Here's how the part is built. I have some questions about the finished solid (model axes, mm). Coordinates: 2 decimals unless noted, no trailing zeros. Order: outer loops, then holes, each group sorted by start corner. A loop starts at its lowest first (then second) coordinate and runs counter-clockwise, first axis right, second up.
```python
from build123d import *

# Parameters (mm, degrees)
SKETCH1_W           = 3.3
SKETCH1_H           = 3
SKETCH1_W_2         = 3
SKETCH1_H_2         = 3.3
BOSS_EXTRUDE1_DEPTH = 3


with BuildPart() as part:
    # Sketch1 → Boss-Extrude1 (new body)
    with BuildSketch(Plane.XY):
        Polygon((165, 252), (156, 243), (120, 243), (111, 252), (111, 288), (120, 297), (156, 297), (165, 288), align=None)
        with Locations((117.15, 254.994383568)):
            Rectangle(SKETCH1_W, SKETCH1_H, mode=Mode.SUBTRACT)
        Polygon((136.5, 274.5), (136.5, 271.5), (133.5, 271.5), (133.5, 268.5), (136.5, 268.5), (136.5, 265.5), (139.5, 265.5), (139.5, 268.5), (142.5, 268.5), (142.5, 271.5), (139.5, 271.5), (139.5, 274.5), align=None, mode=Mode.SUBTRACT)
        with Locations((117.15, 284.994383568)):
            Rectangle(SKETCH1_W, SKETCH1_H, mode=Mode.SUBTRACT)
        with Locations((117.15, 269.994383568)):
            Rectangle(SKETCH1_W, SKETCH1_H, mode=Mode.SUBTRACT)
        with Locations((123.005616432, 249.15)):
            Rectangle(SKETCH1_W_2, SKETCH1_H_2, mode=Mode.SUBTRACT)
        with Locations((158.85, 255.005616432)):
            Rectangle(SKETCH1_W, SKETCH1_H, mode=Mode.SUBTRACT)
        with Locations((152.994383568, 290.85)):
            Rectangle(SKETCH1_W_2, SKETCH1_H_2, mode=Mode.SUBTRACT)
        with Locations((138.005616432, 249.15)):
            Rectangle(SKETCH1_W_2, SKETCH1_H_2, mode=Mode.SUBTRACT)
        with Locations((153.005616432, 249.15)):
            Rectangle(SKETCH1_W_2, SKETCH1_H_2, mode=Mode.SUBTRACT)
        with Locations((158.85, 270.005616432)):
            Rectangle(SKETCH1_W, SKETCH1_H, mode=Mode.SUBTRACT)
        with Locations((158.85, 285.005616432)):
            Rectangle(SKETCH1_W, SKETCH1_H, mode=Mode.SUBTRACT)
        with Locations((137.994383568, 290.85)):
            Rectangle(SKETCH1_W_2, SKETCH1_H_2, mode=Mode.SUBTRACT)
        with Locations((122.994383568, 290.85)):
            Rectangle(SKETCH1_W_2, SKETCH1_H_2, mode=Mode.SUBTRACT)
    extrude(amount=BOSS_EXTRUDE1_DEPTH)


solid = part.part
```
Q1. I need wall thicknesses on L1, parallel to Y at x = 139, z = 2.3; L2, parallel to X at y = 254, z = 1.9; L3, parallel to Y at x = 153, z = 1.8. Which ranges of each line are inside material? Lowest first, please.
Q2. Will these pins go through, and if not, where does the flat tip stop? pin 1 (0.9 mm diameter, centred on y = 248.5, z = 1, fed in from -X); pin 2 (1.5 mm diameter, centred on x = 116.5, z = 1, fed in from -Y).
Q3. If we section it at B-B on z = 0.8: Give the number of separate pieces and of enclosed holes in the cut face, then the cut area to 3 significant figures.
Q4. If we section it at A-A on y = 285: Write out the boundary of the cut face in (x, z), then the cut area to 3 significant figures.
Reply:
1. L1: y = 243 to 247.5, 250.8 to 265.5, 274.5 to 289.2, 292.5 to 297
1. L2: x = 111 to 115.5, 118.8 to 157.2, 160.5 to 165
1. L3: y = 243 to 247.5, 250.8 to 289.2, 292.5 to 297
2. pin 1: stops at x = 114.05
2. pin 2: stops at y = 245.75
3. separate pieces: 1
3. enclosed holes: 13
3. area: 2,590 mm2
4. outline: (111, 0) - (115.5, 0) - (115.5, 3) - (111, 3) - close; (118.8, 0) - (157.2, 0) - (157.2, 3) - (118.8, 3) - close; (160.5, 0) - (165, 0) - (165, 3) - (160.5, 3) - close
4. area: 142 mm2
